Study the drawing (mm; zero at the part's minimum x, y, z) and answer. A direction names the side the tool comes from. Give positions to 0.01 mm unless a question says otherwise; leave off trailing zeros. Loops run counter-clockwise (first coordinate to the right, second up) from the corner with the lowest first, then second, coordinate; pieces in that order, holes last. Notation, with made-up numbers: (56, 65.25) - (106, 65.25) arc R17 ccw to (106, 91.25) - close; hole circle Ø5 at (26.5, -32.5). An arc over 180 degrees is marked (long way). Answer in a Markdown table with one row per item. Add a question column.
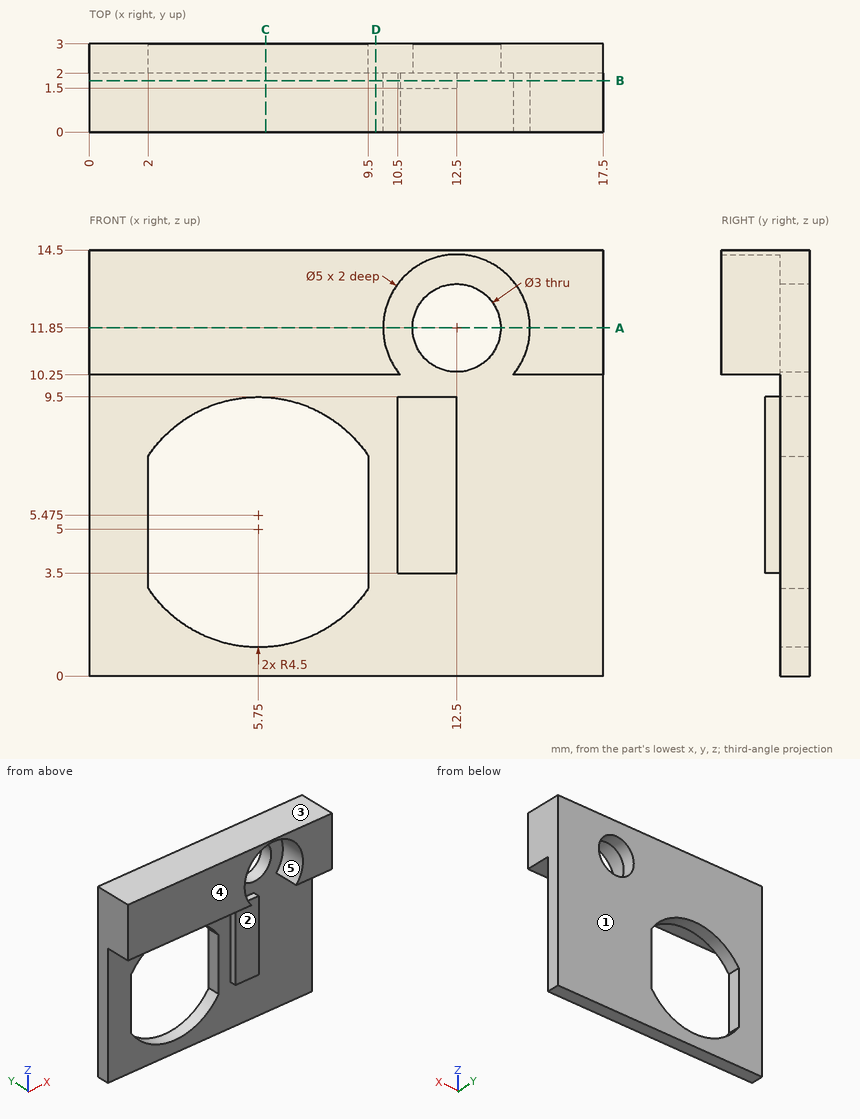
(1) A tool of negligible diameter and unlimited length cuts with its end or side. For the marked faces 1 and 2, from which of +Z, -Z, +X, -X, +Y, -Y can it reach the whole face along a straight path? Write none if from no direction.
(2) A cutting plane is placed at A-A on z = 11.85. Determine the outline of the cut face in (x, y).
(3) Given pin 1 Ø0.6 at (y, z) = (1.5, 5) entering from +X; pin 2 Ø1 at (x, z) = (11.5, 6) entering from -Y; pin 3 Ø0.6 at (x, y) = (11.5, 1.5) entering from -Z; pin 4 Ø4 at (x, z) = (8, 2.5) entering from +Y, each flat-ended and moving along its own axis, determine where each tip first touches the part or whether it passes through.
(4) Find the intervals of material crossed by line 1 along X through (y, z) = (2.35, 11.85); line 2 along X through (y, z) = (2.4, 6); line 3 along Z through (x, y) = (2.5, 1), in increasing order. Write a range as [from, to].
(5) A cutting plane is placed at C-C on x = 6. Determine the outline of the cut face in (y, z).
(6) The mould has two halves that part along Z. Classify the marked faces 3, 4 and 5: pulls with the +Z half, pulls with the -Z half, needs draft (parallel to the pull), parting line crosses it, or undercut.
(7) A cutting plane is placed at B-B on y = 1.75. Determine the outline of the cut face in (x, z).
(8) A cutting plane is placed at D-D on x = 9.75. Determine the outline of the cut face in (y, z).
Evaluation:
| question | item | result |
|---|---|---|
| 1 | face 1 | +Z, -Z, +X, -X, +Y |
| 1 | face 2 | -Z, +X, -X, -Y |
| 2 | outline | (0, 0) - (10, 0) - (10, 2) - (11, 2) - (11, 3) - (0, 3) - close; (14, 2) - (15, 2) - (15, 0) - (17.5, 0) - (17.5, 3) - (14, 3) - close |
| 3 | pin 1 | stops at x = 12.5 |
| 3 | pin 2 | stops at y = 1.5 |
| 3 | pin 3 | stops at z = 3.5 |
| 3 | pin 4 | stops at y = 3 |
| 4 | line 1 | x = [0, 11], [14, 17.5] |
| 4 | line 2 | x = [0, 2], [9.5, 17.5] |
| 4 | line 3 | z = [10.25, 14.5] |
| 5 | outline | (0, 10.25) - (2, 10.25) - (2, 9.49) - (3, 9.49) - (3, 14.5) - (0, 14.5) - close; (2, 0) - (3, 0) - (3, 0.98) - (2, 0.98) - close |
| 6 | face 3 | pulls with the +Z half |
| 6 | face 4 | needs draft |
| 6 | face 5 | undercut |
| 7 | outline | (0, 10.25) - (10.58, 10.25) arc R2.5 cw (long way) to (14.42, 10.25) - (17.5, 10.25) - (17.5, 14.5) - (0, 14.5) - close; (10.5, 3.5) - (12.5, 3.5) - (12.5, 9.5) - (10.5, 9.5) - close |
| 8 | outline | (0, 10.25) - (2, 10.25) - (2, 0) - (3, 0) - (3, 14.5) - (0, 14.5) - close |
